from build123d import *

# Parameters (mm, degrees)
F0_R         = 48.5
F0_R_2       = 43
F1_DEPTH     = 250
F2_DEPTH     = 200
F4_DEPTH     = 70
F5_T2_ANGLE  = 217.5315587112
F5_T4_ANGLE  = 217.5315587112
F5_T8_ANGLE  = 217.5315587112
F5_S9_R      = 43
F5_T10_DEPTH = 60
F5_T14_ANGLE = 217.5315587112
F5_S15_R     = 43
F5_T16_DEPTH = 60


# Not quite as in the source:
# - a fillet or chamfer that OpenCascade refuses, or shapes differently, is made with other operations: its cross-section is extruded or revolved along the edge and cut away or added


with BuildPart() as f1:
    # F0 (on Front) → F1 (new body)
    with BuildSketch(Plane.XZ):
        Circle(F0_R)
        Circle(F0_R_2, mode=Mode.SUBTRACT)
        Circle(F0_R_2)
    extrude(amount=F1_DEPTH)

    # F0 (on Front) → F2 (cut)
    with BuildSketch(Plane.XZ):
        Circle(F0_R)
        Circle(F0_R_2, mode=Mode.SUBTRACT)
    extrude(amount=F2_DEPTH, mode=Mode.SUBTRACT)

    # F3 (on face) → F4 (cut)
    with BuildSketch(Plane.XZ.offset(250)):
        with BuildLine():
            Line((10.3677597397, -47.3788935918), (9.2215594636, 47.6152584899))
            ThreePointArc((9.2215594636, 47.6152584899), (-0.5851588327, 48.4964698627), (-10.3677597397, 47.3788935918))
            Line((-10.3677597397, 47.3788935918), (-9.2215594636, -47.6152584899))
            ThreePointArc((-9.2215594636, -47.6152584899), (0.5851588327, -48.4964698627), (10.3677597397, -47.3788935918))
        make_face()
    extrude(amount=-F4_DEPTH, mode=Mode.SUBTRACT)

    # F5: chamfer of 10 on 4 edges, made by hand

    # F5_s1 → F5_t2 (revolve, cut)
    with BuildSketch(Plane(origin=(0, 0, 0), x_dir=(0, 1, 0), z_dir=(0.9506540069, 0, -0.3102530567))):
        Polygon((-240, 48.5), (-250, 38.5), (-250, 48.5), align=None)
    revolve(axis=Axis((0, -250, 0), (0, -1, 0)), revolution_arc=F5_T2_ANGLE, mode=Mode.SUBTRACT)

    # F5_s3 → F5_t4 (revolve, cut)
    with BuildSketch(Plane(origin=(0, 0, 0), x_dir=(0, 1, 0), z_dir=(-0.9428912961, 0, -0.3331005911))):
        Polygon((-240, -48.5), (-250, -38.5), (-250, -48.5), align=None)
    revolve(axis=Axis((0, -250, 0), (0, 1, 0)), revolution_arc=F5_T4_ANGLE, mode=Mode.SUBTRACT)


with BuildPart() as f5_tool6:
    # F5_s7 → F5_t8 (revolve)
    with BuildSketch(Plane(origin=(0, 0, 0), x_dir=(0, 1, 0), z_dir=(-0.9506540069, 0, 0.3102530567))):
        Polygon((-210, 48.5), (-200, 38.5), (-200, 48.5), align=None)
    revolve(axis=Axis((0, -200, 0), (0, -1, 0)), revolution_arc=F5_T8_ANGLE)

    # F5_s9 → F5_t10 (cut, symmetric)
    with BuildSketch(Plane.XZ.offset(205)):
        Circle(F5_S9_R)
    extrude(amount=F5_T10_DEPTH, both=True, mode=Mode.SUBTRACT)


with BuildPart() as f1_1:
    add(f1.part)

    # F5_t5: cut F5_tool6
    add(f5_tool6.part, mode=Mode.SUBTRACT)


with BuildPart() as f5_tool12:
    # F5_s13 → F5_t14 (revolve)
    with BuildSketch(Plane(origin=(0, 0, 0), x_dir=(0, 1, 0), z_dir=(0.9506540069, 0, -0.3102530567))):
        Polygon((-200, 38.5), (-210, 48.5), (-200, 48.5), align=None)
    revolve(axis=Axis((0, -200, 0), (0, -1, 0)), revolution_arc=F5_T14_ANGLE)

    # F5_s15 → F5_t16 (cut, symmetric)
    with BuildSketch(Plane.XZ.offset(205)):
        Circle(F5_S15_R)
    extrude(amount=F5_T16_DEPTH, both=True, mode=Mode.SUBTRACT)


with BuildPart() as f1_2:
    add(f1_1.part)

    # F5_t11: cut F5_tool12
    add(f5_tool12.part, mode=Mode.SUBTRACT)


solid = f1_2.part
Verification items for the finished model (mm, model axes). Coordinates: 2 decimals unless noted, no trailing zeros. Order: outer loops, then holes, each group sorted by start corner. A loop starts at its lowest first (then second) coordinate and runs counter-clockwise, first axis right, second up.
Item 1: Section check D-D, the plane y = -175.5. Enter the section's corners in (x, z).
Filled in:
outline: circle Ø86 at (0, 0)
Item 2: Depth check by flat-ended pin: pin 1 (3 mm diameter, centred on x = 1.5, z = -3, fed in from -Y); pin 2 (10 mm diameter, centred on y = -156.5, z = 5.5, fed in from -X); pin 3 (6 mm diameter, centred on y = -39, z = -16, fed in from -X); pin 4 (2 mm diameter, centred on x = -30.5, z = 11, fed in from +Y). Enter the tip coordinate at first touch or a pass-through.
Filled in:
pin 1: stops at y = -180
pin 2: stops at x = -43
pin 3: stops at x = -40.99
pin 4: stops at y = 0
Item 3: Section check A-A, the plane y = -227.5. Enter the section's corners in (x, z).
Filled in:
outline: (-10.37, 47.38) arc R48.5 ccw to (-9.22, -47.62) - close; (9.22, 47.62) - (10.37, -47.38) arc R48.5 ccw to start
Item 4: Release check for a two-part mould opening along X. For faces 1 (the face through (-39, -249.5, 0.3)), 2 (the face through (0, -180, 1)), 3 (the face through (-21, -250, 0)) record: +X half, -X half, draft (parallel to the pull), parting line (faces both ways), or undercut.
Filled in:
face 1: -X half
face 2: undercut
face 3: draft
Item 5: Section check B-B, the plane z = 0. Enter the section's corners in (x, y), then the cut area to 3 significant figures.
Filled in:
outline: (-48.5, -240) - (-38.5, -250) - (-9.8, -250) - (-9.8, -180) - (9.8, -180) - (9.8, -250) - (38.5, -250) - (48.5, -240) - (48.5, -210) - (43, -204.5) - (43, 0) - (-43, 0) - (-43, -204.5) - (-48.5, -210) - close
area: 20,500 mm2
Item 6: Material ranges on L1, parallel to Y at x = -3.5, z = -42.5; L2, parallel to X at y = -103.5, z = 1; L3, parallel to X at y = -199.5, z = 5, recorded low to high.
Filled in:
L1: y = -180 to 0
L2: x = -42.99 to 42.99
L3: x = -42.71 to -9.86, 9.74 to 42.71
Item 7: Section check C-C, the plane x = 0. Enter the section's corners in (y, z), then the cut area to 3 significant figures.
Filled in:
outline: (-180, -43) - (0, -43) - (0, 43) - (-180, 43) - close
area: 15,500 mm2
